Check sheet for the modelled part. Datum: model origin and axes. Units: mm. A direction names the side the tool comes from. Coordinates: 2 decimals unless noted, no trailing zeros. Loops run counter-clockwise (first coordinate to the right, second up) from the corner with the lowest first, then second, coordinate; pieces in that order, holes last. Notation, with made-up numbers: (56.5, -35) -> (95.5, -35) arc R16 ccw to (95.5, -4) -> close; hole circle Ø1 at (-25.5, 65.25). An arc over 180 degrees is marked (long way). Use CSV: the item, a comma, the result in double quotes. Start each with the question number.
1. Sectioned sample at B-B, the plane z = -0.5. Record the cut outline in (x, y) (3 decimals).
2. Sectioned sample at C-C, the plane y = 14. Record the cut outline in (x, z) (3 decimals).
3. Thickness scan on L1, parallel to X at y = 17.75, z = -3 (3 decimals); L2, parallel to Y at x = -0.25, z = 3 (3 decimals); L3, parallel to Y at x = 7.05, z = 0 (3 decimals). Record the ranges inside material, lowest first.
4. Set-up check for faces 5 (the face through (6.61, 11.79, 8.424)), 6 (the face through (5, 10, 0)): record each of +Z, -Z, +X, -X, +Y, -Y from which the full face is reachable in a straight line by a thin tool's end or side.
5. Sectioned sample at A-A, the plane y = 18.25. Record the cut outline in (x, z) (3 decimals).
6. Sectioned sample at D-D, the plane x = -7. Record the cut outline in (y, z) (3 decimals).
7. Release check for a two-part mould opening along Z. For faces 1 (the face through (6.61, 11.919, -8.392)), 2 (the face through (-8.175, 8, 0)), 3 (the face through (-6.61, 16.833, 1.344)), 4 (the face through (6.565, 16.833, 1.344)) record: pulls with the +Z half, pulls with the -Z half, needs draft (parallel to the pull), parting line crosses it, or undercut.
8. Gauge pin test, flat ends, axial feed: pin 1 (6 mm diameter, centred on x = -3.5, y = 13, fed in from +Z); pin 2 (8 mm diameter, centred on x = 0.5, z = -2, fed in from +Y) (3 decimals). Record the tip position at first contact, or that the pin passes through.
```python
from build123d import *

# Parameters (mm, degrees)
SKETCH1_W             = 3.175
SKETCH1_H             = 19.05
SKETCH1_W_2           = 10
BOSS_EXTRUDE1_DEPTH   = 3.175
BOSS_EXTRUDE2_START   = 3.175
SKETCH1_3_W           = 3.175
SKETCH1_3_H           = 19.05
BOSS_EXTRUDE2_DEPTH   = 19.05
CUT_EXTRUDE1_DEPTH    = 30.189017626
F_5_0MM_DOWEL_HOLE1_D = 5


with BuildPart() as part:
    # Sketch1 → Boss-Extrude1 (new body)
    with BuildSketch(Plane(origin=(0, 0, 0), x_dir=(1, 0, 0), z_dir=(0, 1, 0))):
        with Locations((-6.5875, 0)):
            Rectangle(SKETCH1_W, SKETCH1_H)
        Rectangle(SKETCH1_W_2, SKETCH1_H)
        with Locations((6.5875, 0)):
            Rectangle(SKETCH1_W, SKETCH1_H)
    extrude(amount=BOSS_EXTRUDE1_DEPTH)

    # Sketch1<3> → Boss-Extrude2 (add)
    with BuildSketch(Plane(origin=(0, 0, 0), x_dir=(1, 0, 0), z_dir=(0, 1, 0)).offset(BOSS_EXTRUDE2_START)):
        with Locations((-6.5875, 0)):
            Rectangle(SKETCH1_3_W, SKETCH1_3_H)
        with Locations((6.5875, 0)):
            Rectangle(SKETCH1_3_W, SKETCH1_3_H)
    extrude(amount=BOSS_EXTRUDE2_DEPTH)

    # Sketch2 → Cut-Extrude1 (cut, through all)
    with BuildSketch(Plane(origin=(8.175, 0, 0), x_dir=(0, 0, -1), z_dir=(1, 0, 0))):
        with BuildLine():
            Line((-9.525, 22.225), (-9.525, 7.225))
            Line((-9.525, 7.225), (-7.290749742, 16.484252172))
            ThreePointArc((-7.290749742, 16.484252172), (-4.6398065, 20.617554255), (0, 22.225))
            Line((0, 22.225), (-9.525, 22.225))
        make_face()
        with BuildLine():
            Line((9.525, 22.225), (0, 22.225))
            ThreePointArc((0, 22.225), (4.6398065, 20.617554255), (7.290749742, 16.484252172))
            Line((7.290749742, 16.484252172), (9.525, 7.225))
            Line((9.525, 7.225), (9.525, 22.225))
        make_face()
    extrude(amount=-CUT_EXTRUDE1_DEPTH, mode=Mode.SUBTRACT)

    # Ø5.0mm Dowel Hole1 (through all)
    with Locations(Plane(origin=(8.175, 0, 0), x_dir=(0, 0, -1), z_dir=(1, 0, 0))):
        with Locations((0, 14.725)):
            Hole(F_5_0MM_DOWEL_HOLE1_D / 2)


solid = part.part
```
Completed:
1,outline,"(-8.175, 0) -> (8.175, 0) -> (8.175, 12.276) -> (5, 12.276) -> (5, 3.175) -> (-5, 3.175) -> (-5, 12.276) -> (-8.175, 12.276) -> close; (-8.175, 17.174) -> (-5, 17.174) -> (-5, 22.208) -> (-8.175, 22.208) -> close; (5, 17.174) -> (8.175, 17.174) -> (8.175, 22.208) -> (5, 22.208) -> close"
2,outline,"(-8.175, -7.89) -> (-5, -7.89) -> (-5, -2.393) -> (-8.175, -2.393) -> close; (-8.175, 2.393) -> (-5, 2.393) -> (-5, 7.89) -> (-8.175, 7.89) -> close; (5, -7.89) -> (8.175, -7.89) -> (8.175, -2.393) -> (5, -2.393) -> close; (5, 2.393) -> (8.175, 2.393) -> (8.175, 7.89) -> (5, 7.89) -> close"
3,L1,"-8.175 to -5, 5 to 8.175"
3,L2,"0 to 3.175"
3,L3,"0 to 12.225, 17.225 to 22.225"
4,face 5,"+Z, +X, -X, +Y"
4,face 6,"+Z, -Z, +Y"
5,outline,"(-8.175, -6.62) -> (-5, -6.62) -> (-5, 6.62) -> (-8.175, 6.62) -> close; (5, -6.62) -> (8.175, -6.62) -> (8.175, 6.62) -> (5, 6.62) -> close"
6,outline,"(0, -9.525) -> (7.225, -9.525) -> (16.484, -7.291) arc R7.5 ccw to (16.484, 7.291) -> (7.225, 9.525) -> (0, 9.525) -> close; hole circle Ø5 at (14.725, 0)"
7,face 1,"pulls with the -Z half"
7,face 2,"needs draft"
7,face 3,"undercut"
7,face 4,"undercut"
8,pin 1,"z = 8.76"
8,pin 2,"y = 3.175"
